from build123d import *

# Parameters (mm, degrees)
SKETCH1_W           = 139.7
SKETCH1_H           = 139.7
BOSS_EXTRUDE1_DEPTH = 6.35
SKETCH4_W           = 139.7
SKETCH4_H           = 139.7
BOSS_EXTRUDE2_DEPTH = 6.35
SHELL1_T            = -6.35
SKETCH5_W           = 127
SKETCH5_H           = 127
BOSS_EXTRUDE4_DEPTH = 12.7
SHELL2_START        = -12.7
SHELL2_OUTLINE_W    = 114.3
SHELL2_OUTLINE_H    = 114.3
SHELL2_DEPTH        = 12.7


# Read off the part's stored shape, not the designer's step: Shell2
with BuildPart() as part:
    # Sketch1 → Boss-Extrude1 (new body)
    with BuildSketch(Plane(origin=(0, 0, 0), x_dir=(1, 0, 0), z_dir=(0, 1, 0))):
        Rectangle(SKETCH1_W, SKETCH1_H)
    extrude(amount=BOSS_EXTRUDE1_DEPTH)

    # Sketch4 → Boss-Extrude2 (add)
    with BuildSketch(Plane(origin=(0, 6.35, 0), x_dir=(1, 0, 0), z_dir=(0, 1, 0))):
        Rectangle(SKETCH4_W, SKETCH4_H)
    extrude(amount=BOSS_EXTRUDE2_DEPTH)

    # Shell1
    shell1_openings = [part.faces().sort_by_distance(p)[0] for p in [
        (0, 12.7, 0),
    ]]
    offset(amount=SHELL1_T, openings=shell1_openings, kind=Kind.INTERSECTION)

    # Sketch5 → Boss-Extrude4 (add)
    with BuildSketch(Plane(origin=(0, 0, 0), x_dir=(-1, 0, 0), z_dir=(0, -1, 0))):
        Rectangle(SKETCH5_W, SKETCH5_H)
    extrude(amount=BOSS_EXTRUDE4_DEPTH)

    # Shell2 outline → Shell2 (cut)
    with BuildSketch(Plane(origin=(0, 0, 0), x_dir=(1, 0, 0), z_dir=(0, 1, 0)).offset(SHELL2_START)):
        Rectangle(SHELL2_OUTLINE_W, SHELL2_OUTLINE_H)
    extrude(amount=SHELL2_DEPTH, mode=Mode.SUBTRACT)


solid = part.part
Part model, mm, in its own coordinate system. A direction names the side the tool comes from. Give positions to 0.01 mm unless a question says otherwise; leave off trailing zeros. Loops run counter-clockwise (first coordinate to the right, second up) from the corner with the lowest first, then second, coordinate; pieces in that order, holes last.
(1) 3-axis set-ups, long thin cutter, end or side, ignore diameter. For faces 5 (the flat face through (-1, 6.35, -1)), 6 (the flat face through (63.5, -6, 1)), 7 (the flat face through (-1, -6, -57.15)), 8 (the flat face through (-63.5, -6, 1)): which of +Z, -Z, +X, -X, +Y, -Y reach the whole face in a straight line?
Return value:
face 5: +Y
face 6: +Z, -Z, +X, -Y
face 7: -Y
face 8: +Z, -Z, -X, -Y
(2) Band-saw the part on A-A (y = 10). Write the cut outline in (x, z).
Return value:
outline: (-69.85, -69.85) - (69.85, -69.85) - (69.85, 69.85) - (-69.85, 69.85) - close; hole (-63.5, -63.5) - (63.5, -63.5) - (63.5, 63.5) - (-63.5, 63.5) - close
(3) Drill centre lines: line 1 along Z through (x, y) = (-23, 7.5); line 2 along Z through (x, y) = (53, -10.5). Where is each one in solid material? Low to high.
Return value:
line 1: z = -69.85 to -63.5, 63.5 to 69.85
line 2: z = -63.5 to -57.15, 57.15 to 63.5
(4) Band-saw the part on B-B (z = -37.5). Write the cut outline in (x, y).
Return value:
outline: (-69.85, 0) - (-63.5, 0) - (-63.5, -12.7) - (-57.15, -12.7) - (-57.15, 0) - (57.15, 0) - (57.15, -12.7) - (63.5, -12.7) - (63.5, 0) - (69.85, 0) - (69.85, 12.7) - (63.5, 12.7) - (63.5, 6.35) - (-63.5, 6.35) - (-63.5, 12.7) - (-69.85, 12.7) - close
(5) Band-saw the part on C-C (x = -5.5). Write the cut outline in (y, z).
Return value:
outline: (-12.7, -63.5) - (0, -63.5) - (0, -69.85) - (12.7, -69.85) - (12.7, -63.5) - (6.35, -63.5) - (6.35, 63.5) - (12.7, 63.5) - (12.7, 69.85) - (0, 69.85) - (0, 63.5) - (-12.7, 63.5) - (-12.7, 57.15) - (0, 57.15) - (0, -57.15) - (-12.7, -57.15) - close
(6) Pull direction Z, two halves, no side cores. Call faces 1 (the flat face through (1, -6, -63.5)), 2 (the flat face through (-6, 12.7, 67)), 3 (the flat face through (-1, 6, 69.85)), 4 (the flat face through (-1, 0, -1)): pulls with the +Z half, pulls with the -Z half, needs draft (parallel to the pull), parting line crosses it, or undercut.
Return value:
face 1: pulls with the -Z half
face 2: needs draft
face 3: pulls with the +Z half
face 4: undercut
(7) Band-saw the part on D-D (y = -2). Write the cut outline in (x, z).
Return value:
outline: (-63.5, -63.5) - (63.5, -63.5) - (63.5, 63.5) - (-63.5, 63.5) - close; hole (-57.15, -57.15) - (57.15, -57.15) - (57.15, 57.15) - (-57.15, 57.15) - close
(8) Pin check, flat tips, straight feed: pin 1 (12 mm diameter, centred on x = -31, y = -9, fed in from -Z); pin 2 (6 mm diameter, centred on x = -45.5, z = 1.5, fed in from +Y); pin 3 (4 mm diameter, centred on x = -23.5, y = -9.5, fed in from +Z). Stop position of each tip, or through.
Return value:
pin 1: stops at z = -63.5
pin 2: stops at y = 6.35
pin 3: stops at z = 63.5
